```python
from build123d import *

# Parameters (mm, degrees)
F0_R     = 10
F1_DEPTH = 25
F2_DEPTH = 25
F4_DEPTH = 35


with BuildPart() as f1:
    # F0 (on Front) → F1 (new body)
    with BuildSketch(Plane.XZ):
        with BuildLine():
            ThreePointArc((-36.9599174113, -9.8680967563), (-35.4426720485, -5.0373667286), (-34.9299123266, 0))
            ThreePointArc((-34.9299123266, 0), (-35.4426720485, 5.0373667286), (-36.9599174113, 9.8680967563))
            ThreePointArc((-36.9599174113, 9.8680967563), (-84.9299123266, 0), (-36.9599174113, -9.8680967563))
        make_face()
        with Locations((-59.9299123266, 0)):
            Circle(F0_R, mode=Mode.SUBTRACT)
        with BuildLine():
            ThreePointArc((-36.9599174113, 9.8680967563), (-35.4426720485, 5.0373667286), (-34.9299123266, 0))
            ThreePointArc((-34.9299123266, 0), (-35.4426720485, -5.0373667286), (-36.9599174113, -9.8680967563))
            Line((-36.9599174113, -9.8680967563), (50.6177291666, -9.8680967563))
            ThreePointArc((50.6177291666, -9.8680967563), (47.5700876734, 0), (50.6177291666, 9.8680967563))
            Line((50.6177291666, 9.8680967563), (-36.9599174113, 9.8680967563))
        make_face()
        with BuildLine():
            ThreePointArc((82.5700876734, 0), (70.2340844845, 16.7207397245), (50.6177291666, 9.8680967563))
            ThreePointArc((50.6177291666, 9.8680967563), (47.5700876734, 0), (50.6177291666, -9.8680967563))
            ThreePointArc((50.6177291666, -9.8680967563), (70.2340844845, -16.7207397245), (82.5700876734, 0))
        make_face()
        with Locations((65.0700876734, 0)):
            Circle(F0_R, mode=Mode.SUBTRACT)
    extrude(amount=F1_DEPTH)

    # F2 (add): a face of the model
    f2_faces = [f1.faces().sort_by_distance(p)[0] for p in [
        (-11.6027124374, -25, 0),
    ]]
    extrude(f2_faces, amount=F2_DEPTH)

    # F3 (on Top) → F4 (intersect, symmetric)
    with BuildSketch(Plane.XY):
        Polygon((82.5700876734, -17.3896358903), (82.5700876734, -2.3896358903), (36.5700876734, -2.3896358903), (-34.9299123266, -28.4135076404), (-84.9299123266, -28.4135076404), (-84.9299123266, -43.4135076404), (-32.285007616, -43.4135076404), (39.214992384, -17.3896358903), align=None)
    extrude(amount=F4_DEPTH, both=True, mode=Mode.INTERSECT)


solid = f1.part
```
The listing builds one solid part. Answer for the finished solid, in the listing's coordinates (mm). A direction names the side the tool comes from. Round coordinates to 2 decimals unless told otherwise and drop trailing zeros. Order: outer loops, then holes, each group sorted by start corner. A loop starts at its lowest first (then second) coordinate and runs counter-clockwise, first axis right, second up. Notation, with made-up numbers: (-38.5, 41.25) -> (-15.5, 41.25) arc R23 cw to (-15.5, 68.25) -> close; hole circle Ø3 at (73.5, 12.25). An arc over 180 degrees is marked (long way). Answer as CSV lines item,"result".
Q1. Which of the six approach directions +Z, -Z, +X, -X, +Y, -Y give full straight-line access (tool end or side, diameter ignored) to faces 1 (the flat face through (7, -23, 9.868)), 2 (the flat face through (-71, -28.414, 0)), 3 (the flat face through (6, -23, -9.868)), 4 (the cylindrical face through (74.308, -9.785, -3.83))?
Computed values:
face 1,"+Z, +Y, -Y"
face 2,"+Z, -Z, -X, +Y"
face 3,"-Z, +Y, -Y"
face 4,"+Y, -Y"
Q2. Consider line 1 (Z direction, x = 2, y = -19); line 2 (Y direction, x = -36, z = -9); line 3 (Y direction, x = 20, z = -2). Determine where each line is inside the solid, lowest interval first. Write a range as from..to.
Computed values:
line 1,"z = -9.87..9.87"
line 2,"y = -43.41..-28.41"
line 3,"y = -24.38..-8.42"
Q3. A cutting plane is placed at A-A on z = 0. Determine the outline of the cut face in (x, y) (1 decimal).
Computed values:
outline,"(-84.9, -43.4) -> (-69.9, -43.4) -> (-69.9, -28.4) -> (-84.9, -28.4) -> close; (-49.9, -43.4) -> (-32.3, -43.4) -> (39.2, -17.4) -> (55.1, -17.4) -> (55.1, -2.4) -> (36.6, -2.4) -> (-34.9, -28.4) -> (-49.9, -28.4) -> close; (75.1, -17.4) -> (82.6, -17.4) -> (82.6, -2.4) -> (75.1, -2.4) -> close"
Q4. Given pin 1 (10 mm diameter, centred on y = -19.5, z = 15.5, fed in from -X); pin 2 (15 mm diameter, centred on x = -63, z = 11, fed in from +Y); pin 3 (12.5 mm diameter, centred on x = 9, y = -20, fed in from -Z), each flat-ended and moving along its own axis, determine where each tip first touches the part or whether it passes through.
Computed values:
pin 1,"stops at x = 51.43"
pin 2,"stops at y = -28.41"
pin 3,"stops at z = -9.87"
Q5. A cutting plane is placed at C-C on y = -32. Determine the outline of the cut face in (x, z).
Computed values:
outline,"(-36.96, -9.87) -> (-0.93, -9.87) -> (-0.93, 9.87) -> (-36.96, 9.87) arc R25 ccw (long way) to start; hole circle Ø20 at (-59.93, 0)"
Q6. For a pull along Z with two mould halves and no side action, classify faces 5 (the cylindrical face through (-50.39, -35.81, 3)), 6 (the flat face through (55.77, -17.39, 4.13)), 7 (the cylindrical face through (82.56, -9.78, -0.62)) as +Z half, -Z half, draft (parallel to the pull), parting line (faces both ways), or undercut.
Computed values:
face 5,"undercut"
face 6,"draft"
face 7,"parting line"
Q7. A cutting plane is placed at B-B on x = -57.5. Determine the outline of the cut face in (y, z).
Computed values:
outline,"(-43.41, -24.88) -> (-28.41, -24.88) -> (-28.41, -9.7) -> (-43.41, -9.7) -> close; (-43.41, 9.7) -> (-28.41, 9.7) -> (-28.41, 24.88) -> (-43.41, 24.88) -> close"
Q8. A cutting plane is placed at D-D on z = 14. Determine the outline of the cut face in (x, y).
Computed values:
outline,"(-80.64, -43.41) -> (-39.22, -43.41) -> (-39.22, -28.41) -> (-80.64, -28.41) -> close; (54.57, -17.39) -> (75.57, -17.39) -> (75.57, -2.39) -> (54.57, -2.39) -> close"
